```python
from build123d import *

# Parameters (mm, degrees)
SKETCH1_W           = 92
SKETCH1_H           = 56
BOSS_EXTRUDE1_DEPTH = 12
SKETCH8_W           = 92
SKETCH8_H           = 2
BOSS_EXTRUDE3_DEPTH = 12
CUT_EXTRUDE1_REACH  = 58.214
SKETCH2_R           = 10.5
CUT_EXTRUDE3_DEPTH  = 6
CUT_EXTRUDE4_REACH  = 57.245
SKETCH6_R           = 2.25
CUT_EXTRUDE5_REACH  = 58.214
FILLET2_R           = 12


with BuildPart() as part:
    # Sketch1 → Boss-Extrude1 (new body)
    with BuildSketch(Plane(origin=(0, 0, 0), x_dir=(1, 0, 0), z_dir=(0, 1, 0))):
        Rectangle(SKETCH1_W, SKETCH1_H)
    extrude(amount=BOSS_EXTRUDE1_DEPTH)

    # Sketch8 → Boss-Extrude3 (add)
    with BuildSketch(Plane(origin=(0, 12, 0), x_dir=(1, 0, 0), z_dir=(0, 1, 0))):
        with Locations((0, 29)):
            Rectangle(SKETCH8_W, SKETCH8_H)
    extrude(amount=-BOSS_EXTRUDE3_DEPTH)

    # Sketch2 → Cut-Extrude1 (cut, up to next)
    with BuildSketch(Plane(origin=(0, 12, 0), x_dir=(1, 0, 0), z_dir=(0, 1, 0)), mode=Mode.PRIVATE) as cut_extrude1_sk1:
        with Locations(Location((-25, -1.5, 0), (0, 0, 270))):
            Circle(SKETCH2_R)
    cut_extrude1_tool1 = extrude(cut_extrude1_sk1.sketch, amount=-CUT_EXTRUDE1_REACH, mode=Mode.PRIVATE) & part.part
    # Sketch2 → Cut-Extrude1 (cut, up to next)
    with BuildSketch(Plane(origin=(0, 12, 0), x_dir=(1, 0, 0), z_dir=(0, 1, 0)), mode=Mode.PRIVATE) as cut_extrude1_sk2:
        with Locations(Location((25, -1.5, 0), (0, 0, 270))):
            Circle(SKETCH2_R)
    cut_extrude1_tool2 = extrude(cut_extrude1_sk2.sketch, amount=-CUT_EXTRUDE1_REACH, mode=Mode.PRIVATE) & part.part
    add(cut_extrude1_tool1.solids().sort_by_distance((-25, 12, 1.5))[0], mode=Mode.SUBTRACT)
    add(cut_extrude1_tool2.solids().sort_by_distance((25, 12, 1.5))[0], mode=Mode.SUBTRACT)

    # Sketch5 → Cut-Extrude3 (cut)
    with BuildSketch(Plane(origin=(0, 12, 0), x_dir=(1, 0, 0), z_dir=(0, 1, 0))):
        with BuildLine():
            Line((-46, -16), (-46, -8.057438524))
            ThreePointArc((-46, -8.057438524), (-46.523662477, 3.053235505), (-41.545392108, 13))
            Line((-41.545392108, 13), (-8.454607892, 13))
            ThreePointArc((-8.454607892, 13), (-3, -1.5), (-8.454607892, -16))
            Line((-8.454607892, -16), (-46, -16))
        make_face()
        with BuildLine():
            Line((46, -16), (46, -8.057438524))
            ThreePointArc((46, -8.057438524), (46.523662477, 3.053235505), (41.545392108, 13))
            Line((41.545392108, 13), (8.454607892, 13))
            ThreePointArc((8.454607892, 13), (3, -1.5), (8.454607892, -16))
            Line((8.454607892, -16), (46, -16))
        make_face()
    extrude(amount=-CUT_EXTRUDE3_DEPTH, mode=Mode.SUBTRACT)

    # Sketch6 → Cut-Extrude4 (cut, up to next)
    with BuildSketch(Plane(origin=(0, 6, 0), x_dir=(1, 0, 0), z_dir=(0, 1, 0)), mode=Mode.PRIVATE) as cut_extrude4_sk1:
        with Locations(Location((-41, -1.5, 0), (0, 0, 270))):
            Circle(SKETCH6_R)
    cut_extrude4_tool1 = extrude(cut_extrude4_sk1.sketch, amount=-CUT_EXTRUDE4_REACH, mode=Mode.PRIVATE) & part.part
    # Sketch6 → Cut-Extrude4 (cut, up to next)
    with BuildSketch(Plane(origin=(0, 6, 0), x_dir=(1, 0, 0), z_dir=(0, 1, 0)), mode=Mode.PRIVATE) as cut_extrude4_sk2:
        with Locations(Location((-9, -1.5, 0), (0, 0, 270))):
            Circle(SKETCH6_R)
    cut_extrude4_tool2 = extrude(cut_extrude4_sk2.sketch, amount=-CUT_EXTRUDE4_REACH, mode=Mode.PRIVATE) & part.part
    # Sketch6 → Cut-Extrude4 (cut, up to next)
    with BuildSketch(Plane(origin=(0, 6, 0), x_dir=(1, 0, 0), z_dir=(0, 1, 0)), mode=Mode.PRIVATE) as cut_extrude4_sk3:
        with Locations(Location((9, -1.5, 0), (0, 0, 270))):
            Circle(SKETCH6_R)
    cut_extrude4_tool3 = extrude(cut_extrude4_sk3.sketch, amount=-CUT_EXTRUDE4_REACH, mode=Mode.PRIVATE) & part.part
    # Sketch6 → Cut-Extrude4 (cut, up to next)
    with BuildSketch(Plane(origin=(0, 6, 0), x_dir=(1, 0, 0), z_dir=(0, 1, 0)), mode=Mode.PRIVATE) as cut_extrude4_sk4:
        with Locations(Location((41, -1.5, 0), (0, 0, 270))):
            Circle(SKETCH6_R)
    cut_extrude4_tool4 = extrude(cut_extrude4_sk4.sketch, amount=-CUT_EXTRUDE4_REACH, mode=Mode.PRIVATE) & part.part
    add(cut_extrude4_tool1.solids().sort_by_distance((-41, 6, 1.5))[0], mode=Mode.SUBTRACT)
    add(cut_extrude4_tool2.solids().sort_by_distance((-9, 6, 1.5))[0], mode=Mode.SUBTRACT)
    add(cut_extrude4_tool3.solids().sort_by_distance((9, 6, 1.5))[0], mode=Mode.SUBTRACT)
    add(cut_extrude4_tool4.solids().sort_by_distance((41, 6, 1.5))[0], mode=Mode.SUBTRACT)

    # Sketch10 → Cut-Extrude5 (cut, up to next)
    with BuildSketch(Plane(origin=(0, 12, 0), x_dir=(1, 0, 0), z_dir=(0, 1, 0)), mode=Mode.PRIVATE) as cut_extrude5_sk1:
        with BuildLine():
            Line((-46, 5.057438524), (-46, 30))
            Line((-46, 30), (-16, 30))
            Line((-16, 30), (-35.667304108, 17.740806196))
            ThreePointArc((-35.667304108, 17.740806196), (-42.056420822, 12.395269294), (-46, 5.057438524))
        make_face()
    cut_extrude5_tool1 = extrude(cut_extrude5_sk1.sketch, amount=-CUT_EXTRUDE5_REACH, mode=Mode.PRIVATE) & part.part
    # Sketch10 → Cut-Extrude5 (cut, up to next)
    with BuildSketch(Plane(origin=(0, 12, 0), x_dir=(1, 0, 0), z_dir=(0, 1, 0)), mode=Mode.PRIVATE) as cut_extrude5_sk2:
        with BuildLine():
            Line((46, 5.057438524), (46, 30))
            Line((46, 30), (16, 30))
            Line((16, 30), (36.615382461, 17.183760068))
            ThreePointArc((36.615382461, 17.183760068), (42.39835371, 11.964668142), (46, 5.057438524))
        make_face()
    cut_extrude5_tool2 = extrude(cut_extrude5_sk2.sketch, amount=-CUT_EXTRUDE5_REACH, mode=Mode.PRIVATE) & part.part
    add(cut_extrude5_tool1.solids().sort_by_distance((-36.403407, 12, -23.114901))[0], mode=Mode.SUBTRACT)
    add(cut_extrude5_tool2.solids().sort_by_distance((36.411287, 12, -23.11647))[0], mode=Mode.SUBTRACT)

    # Fillet2
    fillet2_edges = [part.edges().sort_by_distance(p)[0] for p in [
        (-16, 6, -30),
        (16, 6, -30),
    ]]
    fillet(fillet2_edges, radius=FILLET2_R)


solid = part.part
```
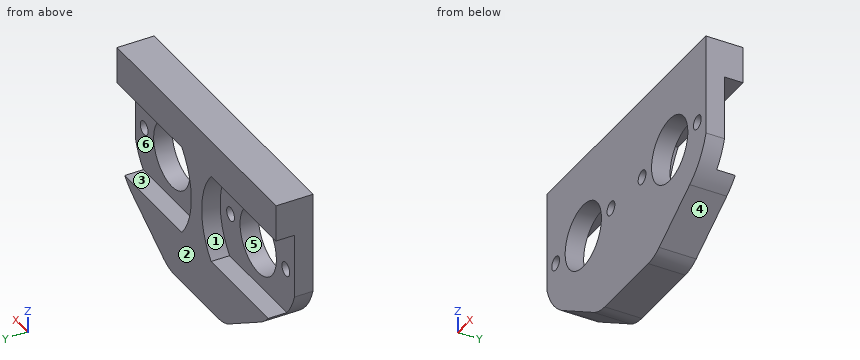
The model under review builds one solid part; all positions refer to its coordinate system, in mm. Face numbers are marked on the shaded views. A direction names the side the tool comes from. Round coordinates to 2 decimals unless told otherwise and drop trailing zeros. Order: outer loops, then holes, each group sorted by start corner. A loop starts at its lowest first (then second) coordinate and runs counter-clockwise, first axis right, second up. Notation, with made-up numbers: M 43,75.5 L 61,75.5 A19 cw 61,92.5 Z; hole C 83.25,-33.75 d11. An arc over 180 degrees is marked long. Use a Markdown table: item, result.
1) Consider section D-D (x = 25). Write out the cut boundary in (y, z).
Report:
| item | result |
|---|---|
| outline | M 0,-24.4 L 12,-24.4 L 12,-13 L 6,-13 L 6,-9 L 0,-9 Z; M 0,12 L 6,12 L 6,16 L 12,16 L 12,28 L 0,28 Z |
2) Wall thickness on line 1 along Y through (x, z) = (-33, -9); line 2 along Z through (x, y) = (33.5, 4.75); line 3 along Z through (x, y) = (-27, 3.75): over which ranges is each line inside the solid? List them lowest first. Write a range as [from, to].
Report:
| item | result |
|---|---|
| line 1 | [0, 6] |
| line 2 | [-19.12, -4.66], [7.66, 28] |
| line 3 | [-23.14, -8.81], [11.81, 28] |
3) Draft analysis for pull direction X (two halves, no side actions). For the marked faces 4, 5 and 6, state which applies: released by +X, released by -X, zero draft, split by the parting line, or undercut.
Report:
| item | result |
|---|---|
| face 4 | released by +X |
| face 5 | undercut |
| face 6 | zero draft |
4) Tool access review of the marked faces 1, 2 and 3: name each direction out of +Z, -Z, +X, -X, +Y, -Y from which nothing blocks a thin tool from reaching the whole face with its end or side.
Report:
| item | result |
|---|---|
| face 1 | -X, +Y |
| face 2 | +Z, -Z, +X, -X, +Y |
| face 3 | +X, +Y |
5) Consider section C-C (y = 7.5). Write out the cut boundary in (x, z), then the cut area to 3 significant figures.
Report:
| item | result |
|---|---|
| outline | M -46,16 L -8.45,16 A22 cw -8.45,-13 L -41.55,-13 A22 ccw -35.67,-17.74 L -18.91,-28.18 A12 ccw -12.57,-30 L 12.57,-30 A12 ccw 18.91,-28.19 L 36.62,-17.18 A22 ccw 41.55,-13 L 8.45,-13 A22 cw 8.45,16 L 46,16 L 46,28 L -46,28 Z |
| area | 2,380 mm^2 |
6) Consider section A-A (z = 1.5). Give the number of separate pieces and of enclosed holes in the cut face, then the cut area to 3 significant figures.
Report:
| item | result |
|---|---|
| separate pieces | 7 |
| enclosed holes | 0 |
| area | 228 mm^2 |
7) Consider section B-B (x = -21.5). Write out the cut boundary in (y, z), then the cut area to 3 significant figures.
Report:
| item | result |
|---|---|
| outline | M 0,-26.57 L 12,-26.57 L 12,-13 L 6,-13 L 6,-8.4 L 0,-8.4 Z; M 0,11.4 L 6,11.4 L 6,16 L 12,16 L 12,28 L 0,28 Z |
| area | 362 mm^2 |
8) Insertion check: pin 1 (8.5 mm diameter, centred on x = -34.5, z = 1, fed in from +Y); pin 2 (4 mm diameter, centred on x = 9, z = 1.5, fed in from -Y); pin 3 (3 mm diameter, centred on x = 28, y = 10, fed in from -Z); pin 4 (1.8 mm diameter, centred on x = -35.5, y = 9, fed in from -Z). Each pin has a flat end and moves straight along its axis. Give the tip position at first contact, or say it passes through.
Report:
| item | result |
|---|---|
| pin 1 | y = 6 |
| pin 2 | through |
| pin 3 | z = -23.47 |
| pin 4 | z = -18.41 |
